For this review, take the finished solid that the model builds, in its own axes (mm). A direction names the side the tool comes from. Give positions to 0.01 mm unless a question says otherwise; leave off trailing zeros. Loops run counter-clockwise (first coordinate to the right, second up) from the corner with the lowest first, then second, coordinate; pieces in that order, holes last. Notation, with made-up numbers: (67.5, 67.5) - (100.5, 67.5) arc R21 ccw to (100.5, 85.5) - close; hole circle Ø1 at (45, 34). An arc over 180 degrees is marked (long way). Answer as CSV lines item,"result".
Autodesk Inventor part; units mm, degrees
ref_plane "YZ Plane" through (0, 0, 0) normal (1, 0, 0) x (0, 1, 0)
ref_plane "XZ Plane" through (0, 0, 0) normal (0, 1, 0) x (-1, 0, 0)
ref_plane "XY Plane" through (0, 0, 0) normal (0, 0, 1) x (1, 0, 0)
sketch "スケッチ1" plane through (0, 0, 0) normal (0, 0, 1) x (1, 0, 0)
  circle A0 centre (0, 0) radius 2.5
  dimension "d0" = 5
extrude "押し出し1" add sketch "スケッチ1" along normal blind 16
sketch "スケッチ2" plane through (0, 0, 0) normal (0, 0, -1) x (-1, 0, 0)
  circle A0 centre (0, 0) radius 5
  dimension "d3" = 10
extrude "押し出し2" add sketch "スケッチ2" along normal blind 2.8
chamfer "面取り1" distance 2.5 angle 45 1 edges at (5, 0, 0)
thread "ねじ1"
sketch "スケッチ3" plane through (0, 0, -2.8) normal (0, 0, -1) x (-1, 0, 0)
  line L0 (1.7321, 0) -> (0.866, -1.5)
  line L1 (0.866, -1.5) -> (-0.866, -1.5)
  line L2 (-0.866, -1.5) -> (-1.7321, 0)
  line L3 (-1.7321, 0) -> (-0.866, 1.5)
  line L4 (-0.866, 1.5) -> (0.866, 1.5)
  line L5 (0.866, 1.5) -> (1.7321, 0)
  point P0 (0, 0)
  point P1 (0, 0)
  dimension "d11" = 3
extrude "押し出し3" cut sketch "スケッチ3" against normal blind 2.5
properties part number "M5皿ネジ　１６" material "鉄 灰色"
1) Consider section B-B on z = 12.25. Write out the cut boundary in (x, y).
From the geometry:
outline,"circle Ø5 at (0, 0)"
2) Insertion check: P1, Ø5, axis at y = 2, z = 3.5, coming from the +X side; P2, Ø3, axis at x = -3.5, z = 13.5, coming from the +Y side; P3, Ø1.9, axis at x = 0, z = -1.5, coming from the -Y side; P4, Ø3, axis at x = 1.5, y = 2.5, coming from the +Z side. Each pin has a flat end and moves straight along its axis. Give the tip position at first contact, or say it passes through.
From the geometry:
P1,"stops at x = 2.5"
P2,"stops at y = 1.5"
P3,"stops at y = -4.95"
P4,"stops at z = 16"
3) Machinability: for faces 4 (the cylindrical face through (-0.54, 2.44, 7.89)), 5 (the flat face through (1.305, 0.74, -1.568)), 6 (the flat face through (0, 0, 16)), which of the approach directions +Z, -Z, +X, -X, +Y, -Y give a long, thin tool a straight path to every point of the face, cutting with its end or side? Answer none if there is none.
From the geometry:
face 4,"+Z"
face 5,"-Z"
face 6,"+Z, +X, -X, +Y, -Y"
4) Draft analysis for pull direction X (two halves, no side actions). For faces 1 (the flat face through (0, -2, -2.8)), 2 (the flat face through (0, -1.5, -2)), 3 (the cylindrical face through (-4.77, -1.5, -2.65)), state which applies: pulls with the +X half, pulls with the -X half, needs draft (parallel to the pull), parting line crosses it, or undercut.
From the geometry:
face 1,"needs draft"
face 2,"undercut"
face 3,"parting line crosses it"
5) Wall thickness on line 1 (Z direction, x = 1, y = 0); line 2 (Z direction, x = -2.5, y = 2.75); line 3 (Y direction, x = -0.75, z = 0.75): over which ranges is each line inside the solid? List them lowest first. Write a range as from..to.
From the geometry:
line 1,"z = -0.3..16"
line 2,"z = -2.8..-1.22"
line 3,"y = -2.38..2.38"
